The listing builds one solid part. Answer for the finished solid, in the listing's coordinates (mm). A direction names the side the tool comes from. Coordinates: 2 decimals unless noted, no trailing zeros. Write each loop counter-clockwise with the first axis right and the second up, starting at its lowest first coordinate (ties: lowest second). Pieces come first, ordered by that corner, then holes.
from build123d import *

# Parameters (mm, degrees)
SKETCH2_W           = 42.15
SKETCH2_H           = 39.52
BOSS_EXTRUDE1_DEPTH = 3
BOSS_EXTRUDE2_DEPTH = 2


with BuildPart() as part:
    # Sketch2 → Boss-Extrude1 (new body)
    with BuildSketch(Plane.XY):
        with Locations((-30.591454667, 0.829849509)):
            Rectangle(SKETCH2_W, SKETCH2_H)
    extrude(amount=BOSS_EXTRUDE1_DEPTH)

    # Sketch3 → Boss-Extrude2 (add)
    with BuildSketch(Plane.XY.offset(3)):
        Polygon((-51.666454667, 9.209849509), (-9.516454667, 9.209849509), (-9.516454667, 12.209849509), (-51.666454667, 12.209849509), (-51.666454667, 10.709849509), align=None)
        Polygon((-51.666454667, 0.829849509), (-51.666454667, -0.670150491), (-9.516454667, -0.670150491), (-9.516454667, 2.329849509), (-51.666454667, 2.329849509), align=None)
        Polygon((-51.666454667, -7.550150491), (-51.666454667, -9.050150491), (-51.666454667, -10.550150491), (-9.516454667, -10.550150491), (-9.516454667, -7.550150491), align=None)
    extrude(amount=BOSS_EXTRUDE2_DEPTH)


solid = part.part
Q1. Which of the six approach directions +Z, -Z, +X, -X, +Y, -Y give full straight-line access (tool end or side, diameter ignored) to faces 5 (the face through (-31, -15, 3)), 6 (the face through (-31, 16, 3)), 7 (the face through (-31, -4, 3)), 8 (the face through (-31, -9, 5))?
Answers below:
face 5: +Z, +X, -X, -Y
face 6: +Z, +X, -X, +Y
face 7: +Z, +X, -X
face 8: +Z, +X, -X, +Y, -Y
Q2. The part is cut by section B-B, the plane y = -11.5. Write down the section's boundary in (x, z), then the cut area to 3 significant figures.
Answers below:
outline: (-51.67, 0) - (-9.52, 0) - (-9.52, 3) - (-51.67, 3) - close
area: 126 mm2
Q3. Determine the mould class of faces 1 (the face through (-30, 12.21, 4)), 2 (the face through (-31, 9.21, 4)), 3 (the face through (-31, 11, 5)), 4 (the face through (-31, -18.93, 1)) for opening direction Y: released by +Y, released by -Y, zero draft, split by the parting line, or undercut.
Answers below:
face 1: released by +Y
face 2: undercut
face 3: zero draft
face 4: released by -Y
Q4. Find the intervals of material crossed by probe 1 along Y at (x, z) = (-26, 4.3); probe 2 along Z at (x, y) = (-14.5, -5.5), in increasing order.
Answers below:
probe 1: y = -10.55 to -7.55, -0.67 to 2.33, 9.21 to 12.21
probe 2: z = 0 to 3
Q5. The part is cut by section A-A, the plane x = -21.5. Write down the section's boundary in (y, z).
Answers below:
outline: (-18.93, 0) - (20.59, 0) - (20.59, 3) - (12.21, 3) - (12.21, 5) - (9.21, 5) - (9.21, 3) - (2.33, 3) - (2.33, 5) - (-0.67, 5) - (-0.67, 3) - (-7.55, 3) - (-7.55, 5) - (-10.55, 5) - (-10.55, 3) - (-18.93, 3) - close
Q6. Given pin 1 (1 mm diameter, centred on x = -40, z = 4, fed in from -Y); pin 2 (7.5 mm diameter, centred on x = -22.5, y = -3, fed in from +Z); pin 3 (1 mm diameter, centred on x = -31.5, z = 4.5, fed in from +Y); pin 4 (2.5 mm diameter, centred on x = -40.5, y = 14.5, fed in from +Z), each flat-ended and moving along its own axis, determine where each tip first touches the part or whether it passes through.
Answers below:
pin 1: stops at y = -10.55
pin 2: stops at z = 5
pin 3: stops at y = 12.21
pin 4: stops at z = 3
